Can you work these out from the drawing? Everything is in mm from the part's minimum corner. A direction names the side the tool comes from. Round coordinates to 2 decimals unless told otherwise and drop trailing zeros. Loops run counter-clockwise (first coordinate to the right, second up) from the corner with the lowest first, then second, coordinate; pieces in that order, holes last. Notation, with made-up numbers: M 16.5,-30 L 22.5,-30 A13 ccw 22.5,-20 Z; hole C 11,48 d6. An arc over 180 degrees is marked long. Use a Markdown table: item, result.
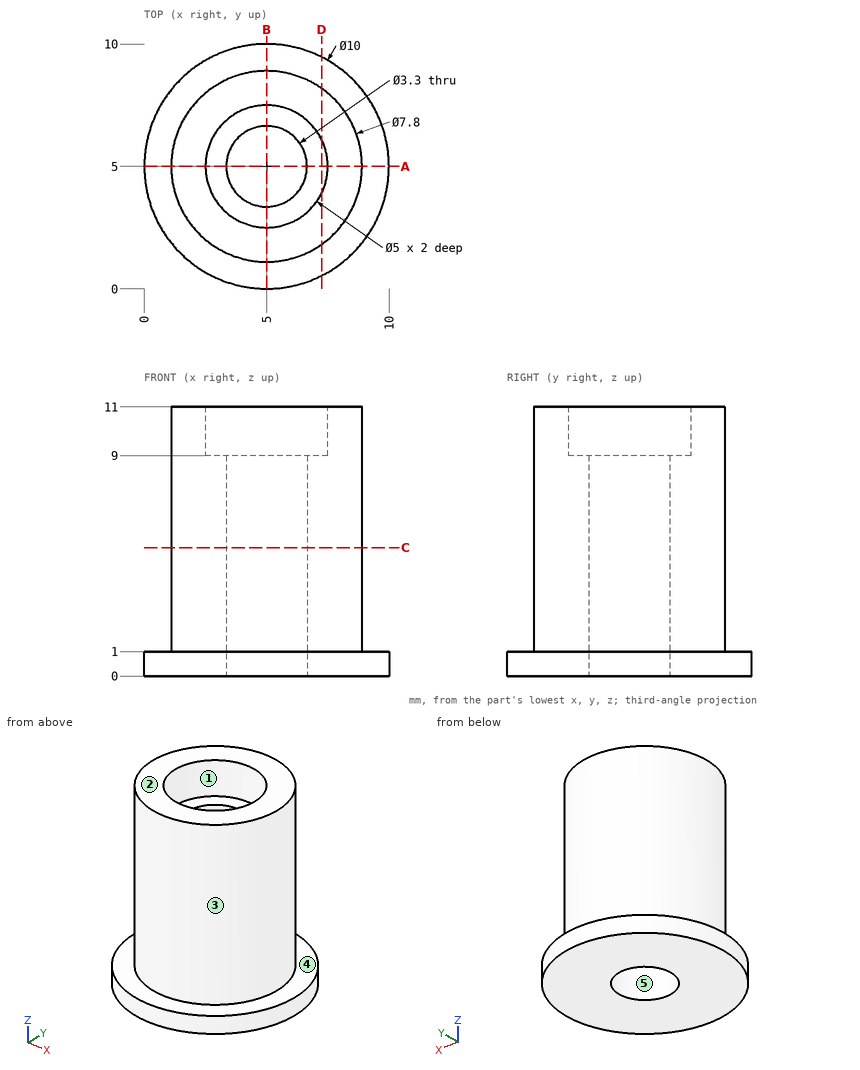
1. Imagine slicing it at C-C, the plane z = 5.25. Write out the boundary of the cut face in (x, y).
Answer sheet:
| item | result |
|---|---|
| outline | C 5,5 d7.8; hole C 5,5 d3.3 |
2. Which directions (+Z, -Z, +X, -X, +Y, -Y) give clear straight access to the entire face, cutting with the end or side of a thin tool? Please do the marked faces 1 and 2.
Answer sheet:
| item | result |
|---|---|
| face 1 | +Z |
| face 2 | +Z, +X, -X, +Y, -Y |
3. I need wall thicknesses on probe 1 along Y at (x, z) = (5, 10.6); probe 2 along Z at (x, y) = (9.25, 5.5); probe 3 along X at (y, z) = (3.75, 3.25). Which ranges of each line are inside material? Lowest first, please. Write a range as from..to.
Answer sheet:
| item | result |
|---|---|
| probe 1 | 1.1..2.5, 7.5..8.9 |
| probe 2 | 0..1 |
| probe 3 | 1.31..3.92, 6.08..8.69 |
4. For pin 1 Ø4 at (x, y) = (8.5, 7) entering from +Z; pin 2 Ø4 at (x, y) = (5, 5) entering from +Z; pin 3 Ø5 at (x, z) = (7.5, 2) entering from -Y; pin 4 Ø3 at (x, z) = (4.5, 7) entering from +Y, each with a flat end and sliding along its axis, tell me the tip position at first contact or that it passes through.
Answer sheet:
| item | result |
|---|---|
| pin 1 | z = 11 |
| pin 2 | z = 9 |
| pin 3 | y = 0 |
| pin 4 | y = 8.9 |
5. Imagine slicing it at A-A, the plane y = 5. Write out the boundary of the cut face in (x, z).
Answer sheet:
| item | result |
|---|---|
| outline | M 0,0 L 3.35,0 L 3.35,9 L 2.5,9 L 2.5,11 L 1.1,11 L 1.1,1 L 0,1 Z; M 6.65,0 L 10,0 L 10,1 L 8.9,1 L 8.9,11 L 7.5,11 L 7.5,9 L 6.65,9 Z |
6. Imagine slicing it at D-D, the plane x = 7.25. Write out the boundary of the cut face in (y, z).
Answer sheet:
| item | result |
|---|---|
| outline | M 0.53,0 L 9.47,0 L 9.47,1 L 8.19,1 L 8.19,11 L 6.09,11 L 6.09,9 L 3.91,9 L 3.91,11 L 1.81,11 L 1.81,1 L 0.53,1 Z |
7. We'd pull the mould along X, two halves only. Please class the marked faces 3, 4 and 5: +X half, -X half, draft (parallel to the pull), parting line (faces both ways), or undercut.
Answer sheet:
| item | result |
|---|---|
| face 3 | parting line |
| face 4 | draft |
| face 5 | undercut |
